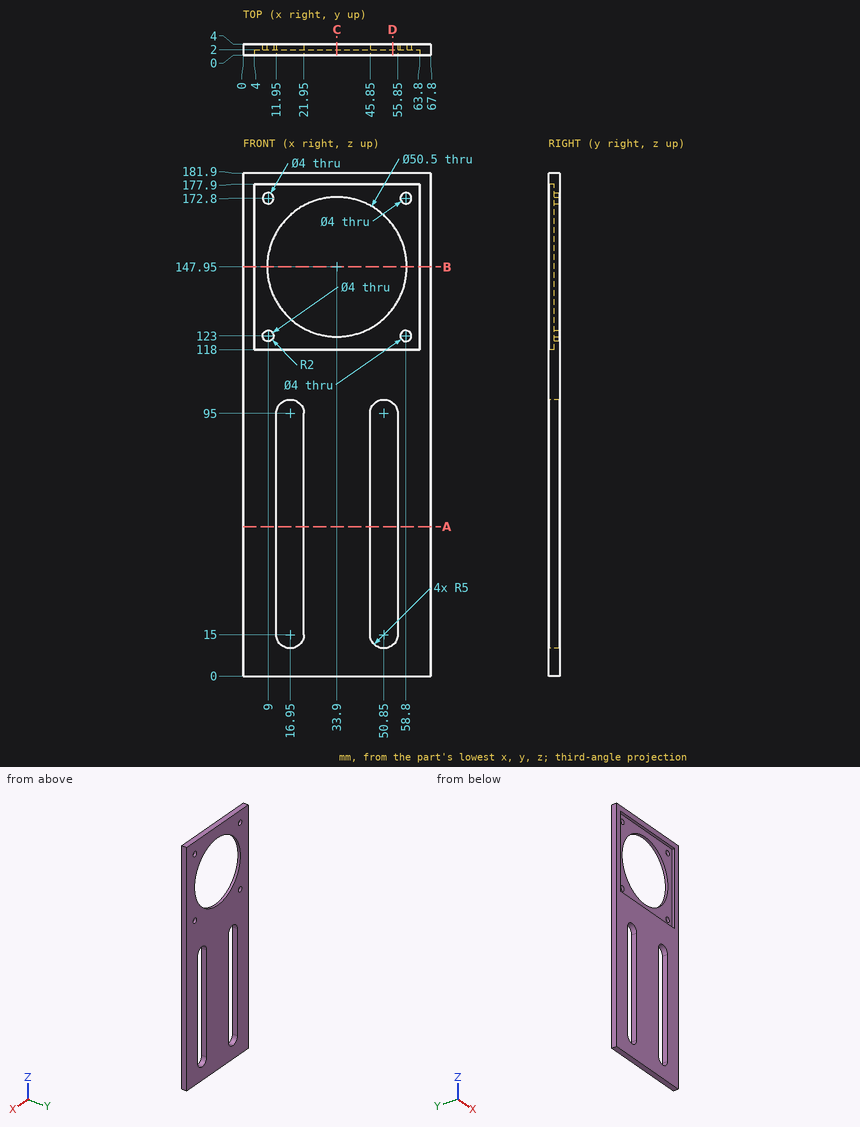
Could you check a few things on this drawing? It's one solid part, dimensions in mm from its lowest x, y, z. Round coordinates to 2 decimals unless told otherwise and drop trailing zeros. Write each loop counter-clockwise with the first axis right and the second up, starting at its lowest first coordinate (ties: lowest second). Pieces come first, ordered by that corner, then holes. Notation, with made-up numbers: (-29, 88.25) -> (20, 88.25) arc R20 cw to (20, 109.25) -> close; hole circle Ø10 at (-28.75, 2). An arc over 180 degrees is marked (long way). Use one line per item in the form item = value. Start each with the question number.
Q1. I'm going to push a flat-ended pin straight in: P1, Ø4.5, axis at x = 9, z = 172.8, coming from the -Y side. Where does the tip first touch, or does it pass through?
Q2. If I drill on probe 1 along X at (y, z) = (2, 93.5); probe 2 along Z at (x, y) = (24, 0.55); probe 3 along X at (y, z) = (1.45, 158), over which ranges is the centre line in solid material (lowest first)? Write a range as [from, to].
Q3. Imagine slicing it at D-D (x = 54). Please give me the cut outline in (y, z), then the cut area to 3 significant figures.
Q4. Imagine slicing it at B-B (z = 147.95). Please give me the cut outline in (x, y).
Q5. Imagine slicing it at A-A (z = 54). Please give me the cut outline in (x, y).
Q6. Imagine slicing it at C-C (x = 33.9). Please give me the cut outline in (y, z).
Worked out:
q1.P1 = 2
q2.probe_1 = [0, 11.95], [21.95, 45.85], [55.85, 67.8]
q2.probe_2 = [0, 118], [177.9, 181.9]
q2.probe_3 = [0, 4], [63.8, 67.8]
q3.outline = (0, 0) -> (4, 0) -> (4, 11.12) -> (0, 11.12) -> close; (0, 98.88) -> (4, 98.88) -> (4, 132.67) -> (2, 132.67) -> (2, 118) -> (0, 118) -> close; (0, 177.9) -> (2, 177.9) -> (2, 163.23) -> (4, 163.23) -> (4, 181.9) -> (0, 181.9) -> close
q3.area = 196 mm^2
q4.outline = (0, 0) -> (4, 0) -> (4, 2) -> (8.65, 2) -> (8.65, 4) -> (0, 4) -> close; (59.15, 2) -> (63.8, 2) -> (63.8, 0) -> (67.8, 0) -> (67.8, 4) -> (59.15, 4) -> close
q5.outline = (0, 0) -> (11.95, 0) -> (11.95, 4) -> (0, 4) -> close; (21.95, 0) -> (45.85, 0) -> (45.85, 4) -> (21.95, 4) -> close; (55.85, 0) -> (67.8, 0) -> (67.8, 4) -> (55.85, 4) -> close
q6.outline = (0, 0) -> (4, 0) -> (4, 122.7) -> (2, 122.7) -> (2, 118) -> (0, 118) -> close; (0, 177.9) -> (2, 177.9) -> (2, 173.2) -> (4, 173.2) -> (4, 181.9) -> (0, 181.9) -> close
